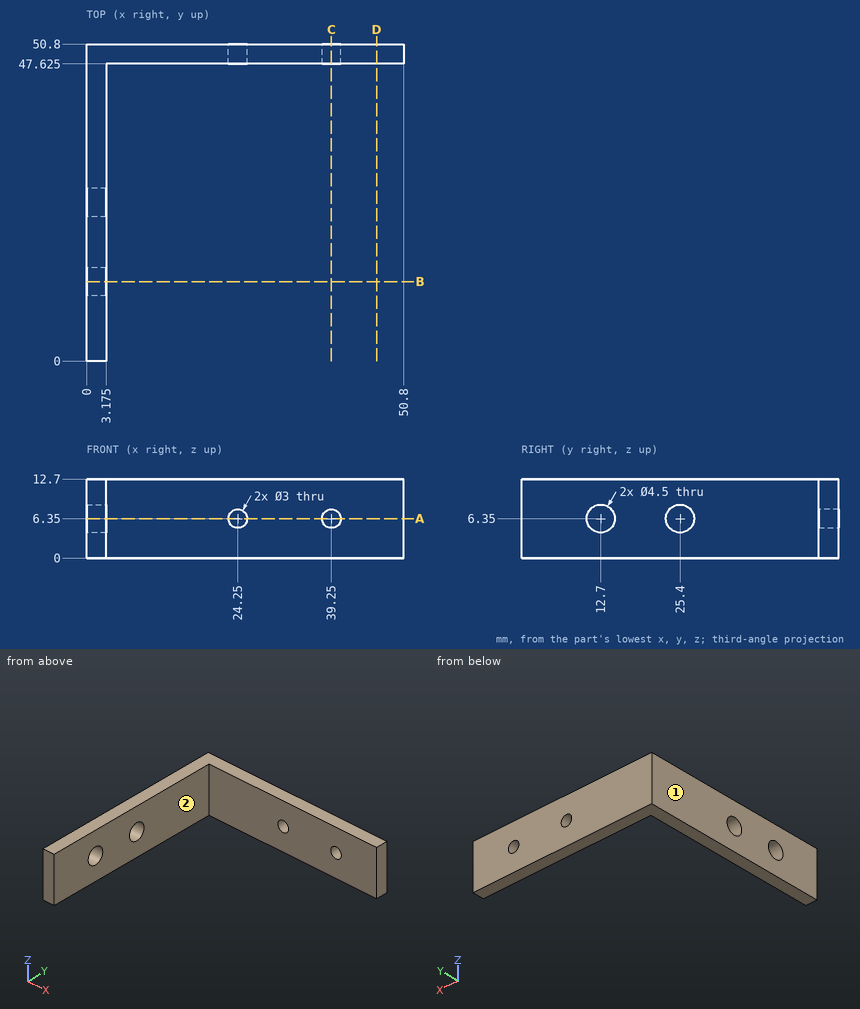
Print and shaded views of the part. All mm, measured from the part's lowest x, y and z. A direction names the side the tool comes from. Round coordinates to 2 decimals unless told otherwise and drop trailing zeros. Write each loop counter-clockwise with the first axis right and the second up, starting at its lowest first coordinate (ties: lowest second). Pieces come first, ordered by that corner, then holes.
(1) Drop flat-ended pins along their axis: P1, Ø1.8, axis at x = 39.25, z = 6.35, coming from the -Y side; P2, Ø6.5, axis at y = 12, z = 9.5, coming from the +X side (3 decimals); P3, Ø3.5, axis at x = 24.25, z = 6.35, coming from the -Y side (3 decimals). Give the stop position or say it passes through.
(2) Slice it at D-D, the plane x = 46.5. Write the cut outline in (y, z) (3 decimals), and give its area (3 significant figures).
(3) Slice it at C-C, the plane x = 39.25. Write the cut outline in (y, z) (3 decimals).
(4) Probe line 1 along Y through (x, z) = (1.2, 6.35); line 2 along X through (y, z) = (49.35, 6.35); line 3 along Y through (x, z) = (46, 8.75) (3 decimals). List the from-to ranges inside material, lowest first.
(5) 3-axis set-ups, long thin cutter, end or side, ignore diameter. For the marked faces 1 and 2: which of +Z, -Z, +X, -X, +Y, -Y reach the whole face in a straight line?
(6) Slice it at B-B, the plane y = 12.7. Write the cut outline in (x, z) (3 decimals), and give its area (3 significant figures).
(7) Slice it at A-A, the plane z = 6.35. Write the cut outline in (x, y) (3 decimals), and give its area (3 significant figures).
From the geometry:
1. P1: passes through
1. P2: stops at x = 3.175
1. P3: stops at y = 47.625
2. outline: (47.625, 0) - (50.8, 0) - (50.8, 12.7) - (47.625, 12.7) - close
2. area: 40.3 mm2
3. outline: (47.625, 0) - (50.8, 0) - (50.8, 4.85) - (47.625, 4.85) - close; (47.625, 7.85) - (50.8, 7.85) - (50.8, 12.7) - (47.625, 12.7) - close
4. line 1: y = 0 to 10.45, 14.95 to 23.15, 27.65 to 50.8
4. line 2: x = 0 to 22.75, 25.75 to 37.75, 40.75 to 50.8
4. line 3: y = 47.625 to 50.8
5. face 1: +Z, -Z, -X, +Y, -Y
5. face 2: +Z, -Z, +X, -Y
6. outline: (0, 0) - (3.175, 0) - (3.175, 4.1) - (0, 4.1) - close; (0, 8.6) - (3.175, 8.6) - (3.175, 12.7) - (0, 12.7) - close
6. area: 26.0 mm2
7. outline: (0, 0) - (3.175, 0) - (3.175, 10.45) - (0, 10.45) - close; (0, 14.95) - (3.175, 14.95) - (3.175, 23.15) - (0, 23.15) - close; (0, 27.65) - (3.175, 27.65) - (3.175, 47.625) - (22.75, 47.625) - (22.75, 50.8) - (0, 50.8) - close; (25.75, 47.625) - (37.75, 47.625) - (37.75, 50.8) - (25.75, 50.8) - close; (40.75, 47.625) - (50.8, 47.625) - (50.8, 50.8) - (40.75, 50.8) - close
7. area: 265 mm2
